Geometry: final body of the model. Coordinates: model frame, mm. A direction names the side the tool comes from. Give positions to 0.01 mm unless a question says otherwise; leave off trailing zeros. Order: outer loops, then holes, each group sorted by start corner. A loop starts at its lowest first (then second) coordinate and runs counter-clockwise, first axis right, second up. Notation, with made-up numbers: (69, 4.25) -> (99, 4.25) arc R31 cw to (99, 43.25) -> close; hole circle Ø10 at (15, 60.5). An arc over 180 degrees is marked (long way). One line per question, with ' | ' between items.
from build123d import *

# Parameters (mm, degrees)
SKIZZE1_R                       = 2
AUFSATZ_LINEAR_AUSTRAGEN1_DEPTH = 5


with BuildPart() as part:
    # Skizze1 → Aufsatz-Linear austragen1 (new body)
    with BuildSketch(Plane(origin=(0, 0, 0), x_dir=(1, 0, 0), z_dir=(0, 1, 0))):
        with BuildLine():
            Line((32.174930969, -0.758710751), (25.406405474, 24.546237926))
            ThreePointArc((25.406405474, 24.546237926), (15.641921228, 31.961749958), (6.033920269, 24.344579298))
            Line((6.033920269, 24.344579298), (4.193711044, 16.842429276))
            Line((4.193711044, 16.842429276), (-18.224781404, 0.973862232))
            ThreePointArc((-18.224781404, 0.973862232), (-21.454022597, -11.53334461), (-9.654845468, -16.790495999))
            Line((-9.654845468, -16.790495999), (8.801061186, -11.423209418))
            Line((8.801061186, -11.423209418), (20.984655174, -13.357550953))
            ThreePointArc((20.984655174, -13.357550953), (30.029331036, -10.12200662), (32.174930969, -0.758710751))
        make_face()
        with Locations(Location((22.552676727, -3.481250613, 0), (0, 0, 270))):
            Circle(SKIZZE1_R, mode=Mode.SUBTRACT)
        with Locations(Location((-12.447323273, -7.188305222, 0), (0, 0, 270))):
            Circle(SKIZZE1_R, mode=Mode.SUBTRACT)
        with Locations(Location((15.746010972, 21.962291706, 0), (0, 0, 270))):
            Circle(SKIZZE1_R, mode=Mode.SUBTRACT)
    extrude(amount=AUFSATZ_LINEAR_AUSTRAGEN1_DEPTH)


solid = part.part
1) Section C-C on z = -21.5. Return loops of the section in (x, y), plus the area to 3 significant figures.
Check result:
outline: (5.34, 0) -> (13.8, 0) -> (13.8, 5) -> (5.34, 5) -> close; (17.69, 0) -> (26.22, 0) -> (26.22, 5) -> (17.69, 5) -> close | area: 85.0 mm^2
2) Material intervals for probe 1 along Z at (x, y) = (23.5, 1.7); probe 2 along Z at (x, y) = (21, 2.75); probe 3 along X at (y, z) = (2.2, 8), sorted ascending. Write a range as from..to.
Check result:
probe 1: z = -28.28..1.72, 5.24..13.44 | probe 2: z = -30.47..2.22, 4.74..13.36 | probe 3: x = -22.41..-14.28, -10.62..31.47
3) Contact query for flat-ended pins moving along their axis: pin 1 Ø10 at (x, z) = (-11.5, -10) entering from +Y; pin 2 Ø1.5 at (x, y) = (27, 1.5) entering from +Z. Output: stop coordinate, or through.
Check result:
pin 1: stops at y = 5 | pin 2: stops at z = 12.77
4) Section A-A on z = 3. Return loops of the section in (x, y).
Check result:
outline: (-21.53, 0) -> (20.61, 0) -> (20.61, 5) -> (-21.53, 5) -> close; (24.49, 0) -> (32.54, 0) -> (32.54, 5) -> (24.49, 5) -> close
5) Section B-B on y = 3.35. Return loops of the section in (x, z), plus the area to 3 significant figures.
Check result:
outline: (-18.22, -0.97) -> (4.19, -16.84) -> (6.03, -24.34) arc R10 ccw to (25.41, -24.55) -> (32.17, 0.76) arc R10 ccw to (20.98, 13.36) -> (8.8, 11.42) -> (-9.65, 16.79) arc R10 ccw to start; hole circle Ø4 at (-12.45, 7.19); hole circle Ø4 at (15.75, -21.96); hole circle Ø4 at (22.55, 3.48) | area: 1,600 mm^2
6) Pull-direction query (X, two-part tool) for faces 3 (the flat face through (28.838, 2.465, -11.717)), 4 (the cylindrical face through (24.239, 2.465, 4.556)), 5 (the flat face through (5.127, 2.465, -20.646)); classes: +X half, -X half, draft (parallel to the pull), parting line (faces both ways), or undercut.
Check result:
face 3: +X half | face 4: undercut | face 5: -X half
7) Set-up query: faces 1 (the flat face through (11, 0, -2)), 2 (the flat face through (14.808, 2.465, 12.377)). Return all of +Z, -Z, +X, -X, +Y, -Y with unobstructed straight access to the full face (end or side cutting, diameter ignored); none if empty.
Check result:
face 1: +Z, -Z, +X, -X, -Y | face 2: +Z, +Y, -Y
8) Section D-D on x = -17. Return loops of the section in (y, z).
Check result:
outline: (0, -1.84) -> (5, -1.84) -> (5, 16.09) -> (0, 16.09) -> close
